Can you work these out from the model? Positions are in its coordinate system, mm. Round coordinates to 2 decimals unless told otherwise and drop trailing zeros. Loops run counter-clockwise (first coordinate to the right, second up) from the corner with the lowest first, then second, coordinate; pieces in that order, holes last.
(1) I want a section at A-A on y = 21. Write out the boundary of the cut face in (x, z) (3 decimals).
(2) I want a section at D-D on y = 77.5. Write out the boundary of the cut face in (x, z) (3 decimals), plus the area to 3 significant figures.
(3) I want a section at B-B on z = 0.95. Write out the boundary of the cut face in (x, y) (3 decimals).
(4) I want a section at C-C on x = 69.5. Write out the boundary of the cut face in (y, z) (3 decimals), plus the area to 3 significant figures.
(5) Will these pins go through, and if not, where does the flat tip stop? pin 1 Ø1 at (y, z) = (-6.5, 2.5) entering from -X; pin 2 Ø1 at (y, z) = (-76.5, 1) entering from +X; pin 3 Ø1 at (x, z) = (23, 2) entering from +Y (3 decimals).
(6) If I drill on line 1 along X through (y, z) = (6, 2.45); line 2 along Y through (x, z) = (-80, 2.45) (3 decimals); line 3 along X through (y, z) = (-58, 0.35), over which ranges is the centre line in solid material (lowest first)?
from build123d import *

# Parameters (mm, degrees)
SKETCH2_W           = 3.175
SKETCH2_H           = 75.333333334
BOSS_EXTRUDE1_DEPTH = 3.175
SKETCH3_W           = 3.175
SKETCH3_H           = 78.508333333
SKETCH3_W_2         = 67.333333334
SKETCH3_H_2         = 3.175
BOSS_EXTRUDE2_DEPTH = 3.175
SKETCH4_W           = 3.175
SKETCH4_H           = 78.508333333
CUT_EXTRUDE1_DEPTH  = 3.175


with BuildPart() as part:
    # Sketch2 → Boss-Extrude1 (new body)
    with BuildSketch(Plane.XY):
        Polygon((-113, 37.666666667), (-113, -37.666666667), (-116.175, -37.666666667), (-116.175, -116.175), (-45.666666667, -116.175), (-45.666666667, -113), (21.666666667, -113), (21.666666667, -116.175), (92.175, -116.175), (92.175, -37.666666667), (95.35, -37.666666667), (95.35, 37.666666667), (92.175, 37.666666667), (92.175, 116.175), (21.666666667, 116.175), (21.666666667, 119.35), (-45.666666667, 119.35), (-45.666666667, 116.175), (-116.175, 116.175), (-116.175, 37.666666667), align=None)
        with Locations((23.254166667, 0)):
            Rectangle(SKETCH2_W, SKETCH2_H, mode=Mode.SUBTRACT)
        with Locations((-47.254166667, 0)):
            Rectangle(SKETCH2_W, SKETCH2_H, mode=Mode.SUBTRACT)
    extrude(amount=BOSS_EXTRUDE1_DEPTH)

    # Sketch3 → Boss-Extrude2 (add)
    with BuildSketch(Plane.XY.offset(3.175)):
        with Locations((-117.7625, 76.920833334)):
            Rectangle(SKETCH3_W, SKETCH3_H)
        with Locations((-117.7625, -76.920833334)):
            Rectangle(SKETCH3_W, SKETCH3_H)
        with Locations((-12, 120.9375)):
            Rectangle(SKETCH3_W_2, SKETCH3_H_2)
    extrude(amount=-BOSS_EXTRUDE2_DEPTH)

    # Sketch4 → Cut-Extrude1 (cut)
    with BuildSketch(Plane.XY.offset(3.175)):
        with Locations((90.5875, 76.920833334)):
            Rectangle(SKETCH4_W, SKETCH4_H)
        with Locations((90.5875, -76.920833334)):
            Rectangle(SKETCH4_W, SKETCH4_H)
    extrude(amount=-CUT_EXTRUDE1_DEPTH, mode=Mode.SUBTRACT)


solid = part.part
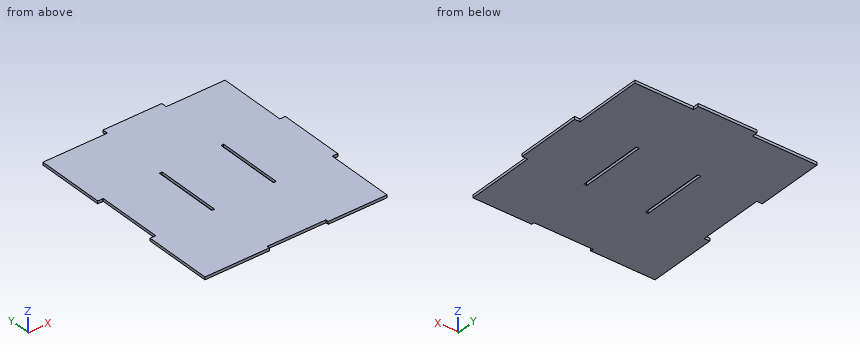
Filled sheet:
1. outline: (-113, 0) - (-48.842, 0) - (-48.842, 3.175) - (-113, 3.175) - close; (-45.667, 0) - (21.667, 0) - (21.667, 3.175) - (-45.667, 3.175) - close; (24.842, 0) - (95.35, 0) - (95.35, 3.175) - (24.842, 3.175) - close
2. outline: (-119.35, 0) - (89, 0) - (89, 3.175) - (-119.35, 3.175) - close
2. area: 662 mm2
3. outline: (-119.35, -116.175) - (-45.667, -116.175) - (-45.667, -113) - (21.667, -113) - (21.667, -116.175) - (89, -116.175) - (89, -37.667) - (95.35, -37.667) - (95.35, 37.667) - (89, 37.667) - (89, 116.175) - (21.667, 116.175) - (21.667, 122.525) - (-45.667, 122.525) - (-45.667, 116.175) - (-119.35, 116.175) - (-119.35, 37.667) - (-113, 37.667) - (-113, -37.667) - (-119.35, -37.667) - close; hole (-48.842, -37.667) - (-45.667, -37.667) - (-45.667, 37.667) - (-48.842, 37.667) - close; hole (21.667, -37.667) - (24.842, -37.667) - (24.842, 37.667) - (21.667, 37.667) - close
4. outline: (-116.175, 0) - (116.175, 0) - (116.175, 3.175) - (-116.175, 3.175) - close
4. area: 738 mm2
5. pin 1: stops at x = -113
5. pin 2: stops at x = 89
5. pin 3: stops at y = 116.175
6. line 1: x = -113 to -48.84, -45.67 to 21.67, 24.84 to 95.35
6. line 2: y = -116.175 to 116.175
6. line 3: x = -119.35 to 89
